Autodesk Inventor part; units mm, degrees
ref_plane "YZ Plane" through (0, 0, 0) normal (1, 0, 0) x (0, 1, 0)
ref_plane "XZ Plane" through (0, 0, 0) normal (0, 1, 0) x (-1, 0, 0)
ref_plane "XY Plane" through (0, 0, 0) normal (0, 0, 1) x (1, 0, 0)
sketch "Sketch5" plane through (0, 0, 0) normal (0, 0, 1) x (1, 0, 0)
  line L0 (1.6002, 0) -> (49.2125, 0)
  line L1 (50.8, 0) -> (50.8, 1.5875)
  line L2 (50.8, 1.5875) -> (0, 1.5875)
  line L3 (0, 1.5875) -> (0, 0)
  line L4 (50.8, 1.5875) -> (49.2125, 1.5875)
  line L5 (49.2125, 0) -> (49.2125, -23.8125)
  line L6 (49.2125, -23.8125) -> (50.8, -23.8125)
  line L7 (50.8, -23.8125) -> (50.8, 1.5875)
  line L8 (49.2125, 0) -> (49.2125, 1.5875)
  line L9 (0, 1.5875) -> (1.6002, 1.5875)
  line L10 (1.6002, 0) -> (1.6002, -23.8125)
  line L11 (1.6002, -23.8125) -> (0, -23.8125)
  line L12 (0, -23.8125) -> (0, 1.5875)
  dimension "d12" = 50.8
  dimension "d13" = 1.5875
  dimension "d14" = 25.4
  dimension "d15" = 1.5875
  dimension "d46" = 1.6002
extrude "Extrusion4" add sketch "Sketch5" along normal blind 50.8
sketch "Sketch6" plane through (50.8, -23.8125, 0) normal (1, 0, 0) x (0, 0, -1)
  line L0 (-50.8, 0) -> (-50.8, 25.4)
  line L1 (-50.8, 25.4) -> (-50.8, 0)
  line L2 (-50.8, 25.4) -> (-48.5778, 0)
  line L3 (-50.8, 23.8125) -> (-50.8, 0)
  line L4 (-48.5778, 0) -> (-50.8, 0)
  line L5 (0, 25.4) -> (-50.8, 25.4)
  point P0 (0, 23.8125)
  dimension "d18" = 85
extrude "Extrusion5" cut sketch "Sketch6" against normal blind 228.6
sketch "Sketch7" plane through (50.8, -23.8125, 0) normal (1, 0, 0) x (0, 0, -1)
  line L0 (0, 0) -> (0, 25.4)
  line L1 (0, 25.4) -> (-50.8, 25.4)
  point P0 (0, 23.8125)
  point P1 (-40.3225, 12.7)
  point P2 (-14.9225, 12.7)
  dimension "d21" = 40.3225
  dimension "d22" = 14.9225
  dimension "d30" = 12.7
  dimension "d31" = 12.7
hole "Hole1" at (50.8, -11.1125, 40.3225) at (50.8, -11.1125, 14.9225) direction (-1, 0, 0) diameter 4.8514 end through all
sketch "Sketch8" plane through (50.8, -23.8125, 0) normal (1, 0, 0) x (0, 0, -1)
  line L0 (0, 0) -> (0, 25.4)
  line L1 (0, 0) -> (0, 25.4)
  line L2 (0, 25.4) -> (0, 0)
  line L3 (-2.2222, 25.4) -> (0, 0)
  line L4 (0, 25.4) -> (-50.8, 25.4)
  line L5 (-2.2222, 25.4) -> (0, 25.4)
  point P0 (0, 23.8125)
  dimension "d32" = 5
extrude "Extrusion6" cut sketch "Sketch8" against normal blind 228.6
sketch "Sketch9" plane through (0, 1.5875, 50.6611) normal (0, -1, 0) x (1, 0, 0)
  line L0 (49.2125, 0) -> (1.6002, 0)
  line L1 (0, -50.6611) -> (0, -2.0833)
  point P0 (12.7, -33.02)
  point P1 (33.02, -12.7)
  dimension "d35" = 12.7
  dimension "d37" = 33.02
  dimension "d47" = 33.02
  dimension "d48" = 12.7
hole "Hole2" at (12.7, 1.5875, 17.6411) at (33.02, 1.5875, 37.9611) direction (0, -1, 0) diameter 4.8514 end through all
properties part number "CAR_039_SweeperBarMount" material "Aluminum 6061"
Geometry: final body of the model. Coordinates: model frame, mm. A direction names the side the tool comes from. Round coordinates to 2 decimals unless told otherwise and drop trailing zeros. Order: outer loops, then holes, each group sorted by start corner. A loop starts at its lowest first (then second) coordinate and runs counter-clockwise, first axis right, second up. Notation, with made-up numbers: (83, 21) - (142, 21) arc R18 cw to (142, 35) - close; hole circle Ø2 at (13.25, 30.5). An arc over 180 degrees is marked (long way). Use CSV: the item, a comma, the result in double quotes. Start each with the question number.
Q1. Access query for faces 1 (the face through (0.79, -8.96, 39.2)), 2 (the face through (1.6, -12, 25)). Directions: +Z, -Z, +X, -X, +Y, -Y. A direction counts if a zero-diameter tool reaches every point of the face in a straight line with its end or side. Return the directions, or none.
Q2. Section query D-D (z = 18). Return loops of the section in (x, y), and give its area (3 significant figures).
Q3. Material intervals for line 1 along X through (y, z) = (-11.25, 6); line 2 along Y through (x, z) = (18.5, 41.5); line 3 along Z through (x, y) = (33.02, 0.85), sorted ascending. Write a range as from..to.
Q4. First-contact query: pin 1 (12 mm diameter, centred on x = 20, z = 19, fed in from -Y); pin 2 (1 mm diameter, centred on y = -2, z = 36, fed in from -X). Flat tips, straight axial feed; report the tip coordinate or a pass-through.
Q5. Section query C-C (y = -2.5). Return loops of the section in (x, z), and give its area (3 significant figures).
Q6. Mould query, pull axis X, two halves, no side actions, for faces 3 (the face through (50.8, -11, 25)), 4 (the face through (26, 1.588, 26)), 5 (the face through (25, 0, 26)), 6 (the face through (0, -11, 25)). Classes: +X half, -X half, draft (parallel to the pull), parting line (faces both ways), or undercut.
Q7. Section query B-B (z = 44.5). Return loops of the section in (x, y), and give its area (3 significant figures).
Q8. Section query A-A (x = 12.7). Return loops of the section in (y, z).
Result set:
1,face 1,"+X, -X"
1,face 2,"+Z, -Z, -Y"
2,outline,"(0, -23.81) - (1.6, -23.81) - (1.6, 0) - (10.3, 0) - (10.3, 1.59) - (0, 1.59) - close; (15.1, 0) - (49.21, 0) - (49.21, -23.81) - (50.8, -23.81) - (50.8, 1.59) - (15.1, 1.59) - close"
2,area,"149 mm2"
3,line 1,"x = 0..1.6, 49.21..50.8"
3,line 2,"y = 0..1.59"
3,line 3,"z = 2.16..35.54, 40.39..50.74"
4,pin 1,"stops at y = 0"
4,pin 2,"stops at x = 0"
5,outline,"(0, 1.86) - (1.6, 1.86) - (1.6, 50.44) - (0, 50.44) - close; (49.21, 1.86) - (50.8, 1.86) - (50.8, 50.44) - (49.21, 50.44) - close"
5,area,"155 mm2"
6,face 3,"+X half"
6,face 4,"draft"
6,face 5,"undercut"
6,face 6,"-X half"
7,outline,"(0, -23.81) - (1.6, -23.81) - (1.6, 0) - (49.21, 0) - (49.21, -23.81) - (50.8, -23.81) - (50.8, 1.59) - (0, 1.59) - close"
7,area,"157 mm2"
8,outline,"(0, 2.08) - (1.59, 2.22) - (1.59, 15.22) - (0, 15.22) - close; (0, 20.07) - (1.59, 20.07) - (1.59, 50.8) - (0, 50.66) - close"
